Design review of the part built by this model. Coordinates are the model's own, in mm. Coordinates: 2 decimals unless noted, no trailing zeros. Loops run counter-clockwise (first coordinate to the right, second up) from the corner with the lowest first, then second, coordinate; pieces in that order, holes last. Notation, with made-up numbers: (-17, -5.75) -> (23, -5.75) arc R31 cw to (23, 25.25) -> close; hole circle Ø4 at (83.5, 44.5). An arc over 180 degrees is marked (long way). Answer as a JSON object with one key per item and string values.
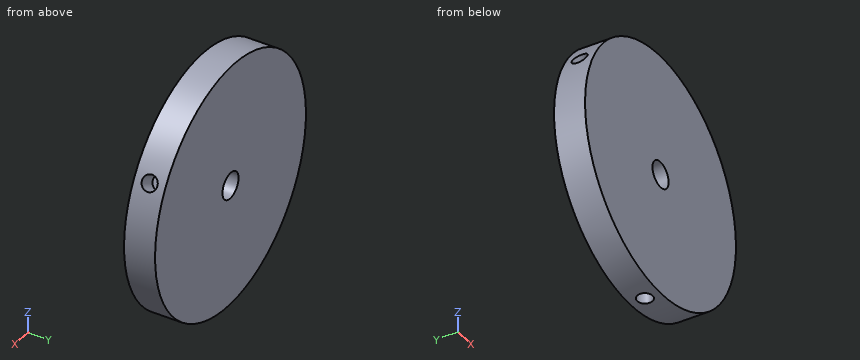
```python
from build123d import *

# Parameters (mm, degrees)
SKETCH1_R           = 38.1508
BOSS_EXTRUDE1_DEPTH = 9.525
SKETCH4_R           = 2.3749
CUT_EXTRUDE2_DEPTH  = 6.35
CIRPATTERN1_COUNT   = 3
SKETCH6_R           = 4.064
CUT_EXTRUDE4_DEPTH  = 55.787705952


with BuildPart() as part:
    # Sketch1 → Boss-Extrude1 (new body)
    with BuildSketch(Plane(origin=(0, 0, 0), x_dir=(1, 0, 0), z_dir=(0, 1, 0))):
        with Locations(Location((0, 0, 0), (0, 0, 90))):
            Circle(SKETCH1_R)
    extrude(amount=BOSS_EXTRUDE1_DEPTH)

    # Sketch4 → Cut-Extrude2 (cut)
    with BuildSketch(Plane(origin=(-33.039561975, 0, 19.0754), x_dir=(0, -1, 0), z_dir=(-0.8660254037844433, 0, 0.49999999999999195))):
        with Locations(Location((-4.7625, 0, 0), (0, 0, 90))):
            Circle(SKETCH4_R)
    cut_extrude2 = extrude(amount=-CUT_EXTRUDE2_DEPTH, mode=Mode.SUBTRACT)

    # CirPattern1: Cut-Extrude2 ×3 about axis
    cirpattern1_axis = Axis((0, 0, 0), (0, 1, 0))
    for i in range(1, CIRPATTERN1_COUNT):
        add(cut_extrude2.rotate(cirpattern1_axis, i * 360 / CIRPATTERN1_COUNT), mode=Mode.SUBTRACT)

    # Sketch6 → Cut-Extrude4 (cut, through all)
    with BuildSketch(Plane(origin=(0, 9.525, 0), x_dir=(1, 0, 0), z_dir=(0, 1, 0))):
        with Locations(Location((0, 0, 0), (0, 0, 270))):
            Circle(SKETCH6_R)
    extrude(amount=-CUT_EXTRUDE4_DEPTH, mode=Mode.SUBTRACT)


solid = part.part
```
1) Wall thickness on probe 1 along Y at (x, z) = (-31, 18) (3 decimals); probe 2 along X at (y, z) = (5, 0); probe 3 along Z at (x, y) = (1, 1.25): over which ranges is each line inside the solid? List them lowest first.
Completed:
{"probe 1": "0 to 2.389, 7.136 to 9.525", "probe 2": "-38.15 to -4.06, 4.06 to 38.15", "probe 3": "-38.14 to -3.94, 3.94 to 38.14"}
2) Add section D-D, the plane x = 25. Give the boundary of the cut face in (y, z) (3 decimals).
Completed:
{"outline": "(0, -28.818) -> (9.525, -28.818) -> (9.525, 28.818) -> (0, 28.818) -> close"}
3) Clearance check with flat-ended pins moving along their axes: pin 1 Ø2 at (x, y) = (-28, 7.5) entering from -Z; pin 2 Ø2 at (y, z) = (2, -24) entering from +X; pin 3 Ø3 at (y, z) = (8, -12.5) entering from +X; pin 4 Ø6 at (x, z) = (26, -11) entering from -Y. State where each tip first meets the part, or that it passes through.
Completed:
{"pin 1": "z = -26.95", "pin 2": "x = 30.44", "pin 3": "x = 36.53", "pin 4": "y = 0"}
4) Add section B-B, the plane x = 0. Give the boundary of the cut face in (y, z) (3 decimals).
Completed:
{"outline": "(0, -38.151) -> (2.388, -38.151) -> (2.388, -31.801) -> (7.137, -31.801) -> (7.137, -38.151) -> (9.525, -38.151) -> (9.525, -4.064) -> (0, -4.064) -> close; (0, 4.064) -> (9.525, 4.064) -> (9.525, 38.151) -> (0, 38.151) -> close"}
5) Add section C-C, the plane y = 5.75. Give the boundary of the cut face in (x, z).
Completed:
{"outline": "(-34.07, 17.17) arc R38.15 ccw to (-2.16, -38.09) -> (-2.16, -31.8) -> (2.16, -31.8) -> (2.16, -38.09) arc R38.15 ccw to (34.07, 17.17) -> (28.62, 14.03) -> (26.46, 17.77) -> (31.91, 20.92) arc R38.15 ccw to (-31.91, 20.92) -> (-26.46, 17.77) -> (-28.62, 14.03) -> close; hole circle Ø8.13 at (0, 0)"}
6) Add section A-A, the plane z = 0. Give the boundary of the cut face in (x, y) (3 decimals), and give its area (3 significant figures).
Completed:
{"outline": "(-38.151, 0) -> (-4.064, 0) -> (-4.064, 9.525) -> (-38.151, 9.525) -> close; (4.064, 0) -> (38.151, 0) -> (38.151, 9.525) -> (4.064, 9.525) -> close", "area": "649 mm²"}
